Can you work these out from the drawing? Everything is in mm from the part's minimum corner. Coordinates: 2 decimals unless noted, no trailing zeros. Write each loop counter-clockwise with the first axis right and the second up, starting at its lowest first coordinate (ties: lowest second). Pieces come first, ordered by that corner, then holes.
(1) Imagine slicing it at A-A, the plane x = 60. List the corners of the cut face in (y, z) for me.
(2) For pin 1 Ø1.5 at (y, z) = (30, 2.5) entering from -X, with a flat end and sliding along its axis, tell me the tip position at first contact or that it passes through.
(3) Please list where these lines run through material, in increasing order: probe 1 along Y at (x, z) = (60, 1.6); probe 2 along X at (y, z) = (28, 0.9); probe 3 along Y at (x, z) = (59.5, 0.25).
(4) Imagine slicing it at B-B, the plane z = 2.15. List the corners of the cut face in (x, y) for me, plus the area to 3 significant figures.
(5) Imagine slicing it at C-C, the plane y = 7.5. List the corners of the cut face in (x, z) for me.
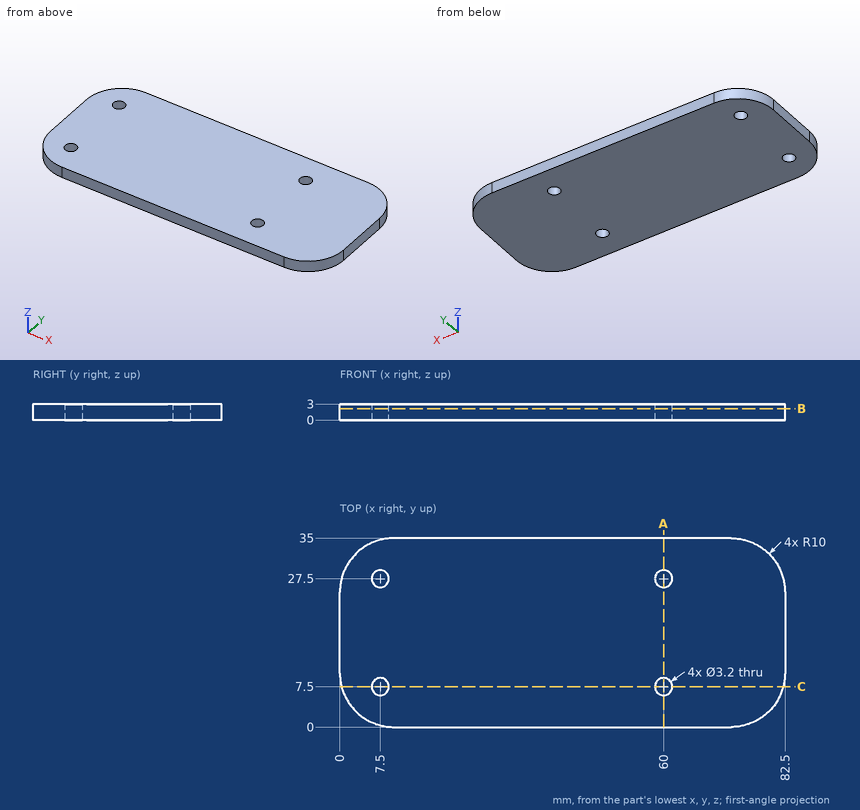
Recorded:
1. outline: (0, 0) - (5.9, 0) - (5.9, 3) - (0, 3) - close; (9.1, 0) - (25.9, 0) - (25.9, 3) - (9.1, 3) - close; (29.1, 0) - (35, 0) - (35, 3) - (29.1, 3) - close
2. pin 1: stops at x = 0.95
3. probe 1: y = 0 to 5.9, 9.1 to 25.9, 29.1 to 35
3. probe 2: x = 0.46 to 5.98, 9.02 to 58.48, 61.52 to 82.04
3. probe 3: y = 0 to 5.98, 9.02 to 25.98, 29.02 to 35
4. outline: (0, 10) arc R10 ccw to (10, 0) - (72.5, 0) arc R10 ccw to (82.5, 10) - (82.5, 25) arc R10 ccw to (72.5, 35) - (10, 35) arc R10 ccw to (0, 25) - close; hole circle Ø3.2 at (7.5, 7.5); hole circle Ø3.2 at (7.5, 27.5); hole circle Ø3.2 at (60, 7.5); hole circle Ø3.2 at (60, 27.5)
4. area: 2,770 mm2
5. outline: (0.32, 0) - (5.9, 0) - (5.9, 3) - (0.32, 3) - close; (9.1, 0) - (58.4, 0) - (58.4, 3) - (9.1, 3) - close; (61.6, 0) - (82.18, 0) - (82.18, 3) - (61.6, 3) - close
